Read the model definition and answer for the solid it produces. Units are mm, in the model's axes. Round coordinates to 2 decimals unless told otherwise and drop trailing zeros. Loops run counter-clockwise (first coordinate to the right, second up) from the corner with the lowest first, then second, coordinate; pieces in that order, holes last. Notation, with made-up numbers: M 37,-17.5 L 80,-17.5 A23 cw 80,21.5 Z; hole C -11.5,25 d4. An arc over 180 degrees is marked long. Write each question's results on one line, items separated by ' | '.
from build123d import *

# Parameters (mm, degrees)
F1_DEPTH = 381
F2_R     = 25.4
F3_R     = 1.27


with BuildPart() as f1:
    # F0 (on Front) → F1 (new body, symmetric)
    with BuildSketch(Plane.XZ):
        with BuildLine():
            ThreePointArc((38.1, 41.6392), (-3.574456, 16.768836), (-50.8, 5.586557))
            Line((-50.8, 5.586557), (-63.5, 0))
            ThreePointArc((-63.5, 0), (4.891593, 13.171017), (63.5, 50.8))
            Line((63.5, 50.8), (38.1, 41.6392))
        make_face()
    extrude(amount=F1_DEPTH, both=True)

    # F2
    f2_edges = [f1.edges().sort_by_distance(p)[0] for p in [
        (38.1, 0, 41.6392),
        (-50.8, 0, 5.586557),
    ]]
    fillet(f2_edges, radius=F2_R)

    # F3
    f3_edges = [f1.edges().sort_by_distance(p)[0] for p in [
        (-63.5, 0, 0),
        (63.5, 0, 50.8),
    ]]
    fillet(f3_edges, radius=F3_R)


solid = f1.part
Item 1: The part is cut by section B-B (z = 21.5). Determine the outline of the cut face in (x, y).
Outcome:
outline: M 6.98,-381 L 22.85,-381 L 22.85,381 L 6.98,381 Z
Item 2: Straight lines are drawn through the part: line 1 (Z direction, x = 30, y = -339); line 2 (X direction, y = 346.5, z = 38); line 3 (Z direction, x = 35, y = 70). For each, find the intervals that lie inside material, in ascending order.
Outcome:
line 1: z = 25.5 to 35.37 | line 2: x = 33.53 to 48.53 | line 3: z = 28.56 to 39.14
Item 3: The part is cut by section A-A (y = 247). Determine the outline of the cut face in (x, z).
Outcome:
outline: M -57.72,2.54 A1.27 ccw -57.17,0.11 A184.15 ccw 58.85,46.52 A1.27 ccw 57.57,48.66 L 42.1,43.08 A25.4 ccw 35.02,39.16 A159.46 cw -46.98,5.94 A25.4 ccw -54.58,3.92 Z
Item 4: Flat-ended cylindrical pins translate along their axes: pin 1 (4 mm diameter, centred on x = 44.5, y = 112.5, fed in from +Z); pin 2 (3 mm diameter, centred on x = 13, z = 26, fed in from -Y); pin 3 (6 mm diameter, centred on x = 44.5, y = -56, fed in from -Z); pin 4 (1.5 mm diameter, centred on x = -2.5, y = 127, fed in from -Z). Find the tip coordinate at first contact, or state that the pin passes through.
Outcome:
pin 1: stops at z = 44.67 | pin 2: stops at y = -381 | pin 3: stops at z = 32.87 | pin 4: stops at z = 10.14
Item 5: The part is cut by section C-C (x = -14). Determine the outline of the cut face in (y, z), plus the area to 3 significant figures.
Outcome:
outline: M -381,6.78 L 381,6.78 L 381,12.96 L -381,12.96 Z | area: 4,710 mm2
